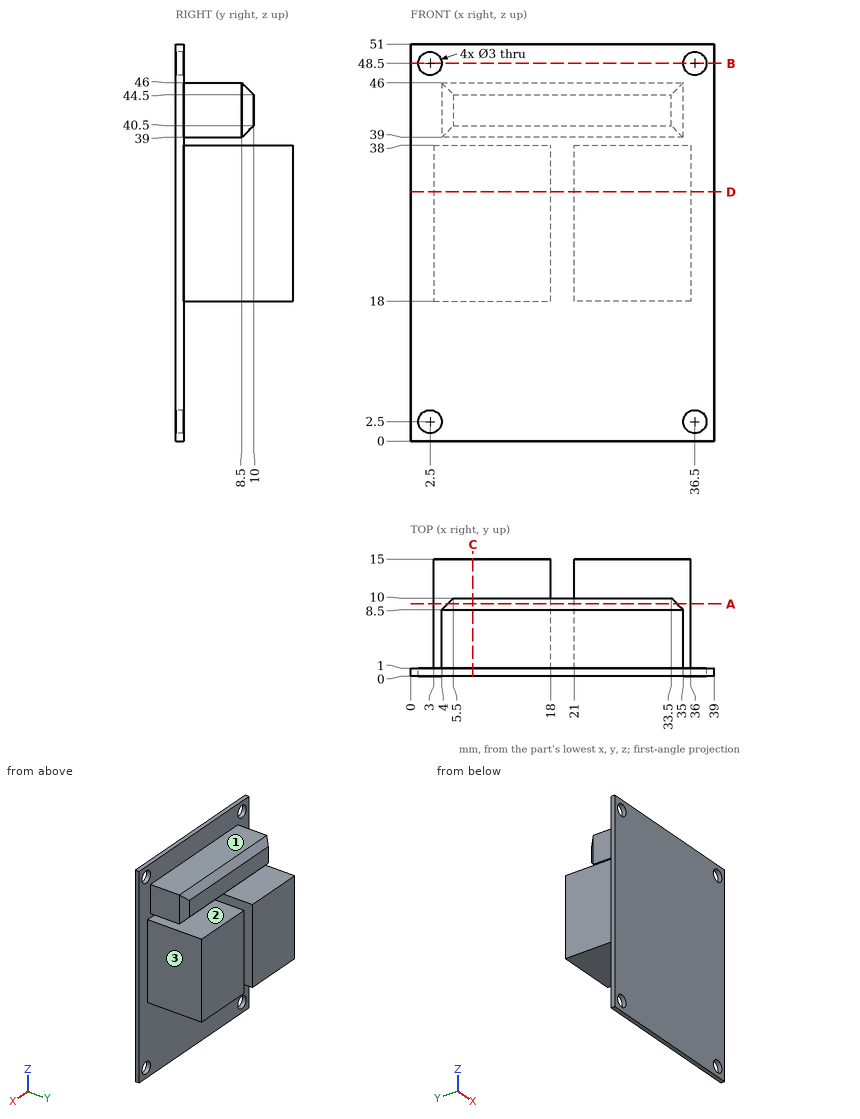
Study the drawing (mm; zero at the part's minimum x, y, z) and answer. A direction names the side the tool comes from. Give positions to 0.01 mm unless a question says otherwise; leave off trailing zeros. Loops run counter-clockwise (first coordinate to the right, second up) from the corner with the lowest first, then second, coordinate; pieces in that order, holes last. Notation, with made-up numbers: M -18.75,89 L 33.25,89 A23 ccw 33.25,114 Z; hole C 21,72.25 d8. An arc over 180 degrees is marked long. One line per item, written item: value. Start each with the question number.
1. Each of these flat-tipped pins is pushed along its axis until it touches: P1, Ø1.5, axis at y = 9.5, z = 26.5, coming from the +X side; P2, Ø4, axis at x = 21, y = 4, coming from the +Z side; P3, Ø3, axis at x = 5.5, y = 5.5, coming from the -Z side. Where does it stop, or does it pass through?
2. Find section A-A (y = 9.25). Give the vertices of the cut face in (x, z), and give its area (3 significant figures).
3. Find section D-D (z = 32). Give the vertices of the cut face in (x, y), and give its area (3 significant figures).
4. Find section B-B (z = 48.5). Give the vertices of the cut face in (x, y), and give its area (3 significant figures).
5. Find section C-C (x = 8). Give the vertices of the cut face in (y, z).
6. Find the intervals of material crossed by probe 1 along Z at (x, y) = (2.5, 0.75); probe 2 along Z at (x, y) = (22.5, 2.5); probe 3 along X at (y, z) = (13.5, 34.5), in increasing order.
7. Which of the six approach directions +Z, -Z, +X, -X, +Y, -Y give full straight-line access (tool end or side, diameter ignored) to the marked faces 1, 2 and 3?
Reported:
1. P1: stops at x = 36
1. P2: stops at z = 46
1. P3: stops at z = 18
2. outline: M 3,18 L 18,18 L 18,38 L 3,38 Z; M 4.75,39.75 L 34.25,39.75 L 34.25,45.25 L 4.75,45.25 Z; M 21,18 L 36,18 L 36,38 L 21,38 Z
2. area: 762 mm²
3. outline: M 0,0 L 39,0 L 39,1 L 36,1 L 36,15 L 21,15 L 21,1 L 18,1 L 18,15 L 3,15 L 3,1 L 0,1 Z
3. area: 459 mm²
4. outline: M 0,0 L 1,0 L 1,1 L 0,1 Z; M 4,0 L 35,0 L 35,1 L 4,1 Z; M 38,0 L 39,0 L 39,1 L 38,1 Z
4. area: 33.0 mm²
5. outline: M 0,0 L 1,0 L 1,18 L 15,18 L 15,38 L 1,38 L 1,39 L 8.5,39 L 10,40.5 L 10,44.5 L 8.5,46 L 1,46 L 1,51 L 0,51 Z
6. probe 1: z = 0 to 1, 4 to 47, 50 to 51
6. probe 2: z = 18 to 38, 39 to 46
6. probe 3: x = 3 to 18, 21 to 36
7. face 1: +Z, +X, -X, +Y
7. face 2: +X, -X, +Y
7. face 3: +Z, -Z, +X, +Y
